```python
from build123d import *

# Parameters (mm, degrees)
SKETCH1_W              = 44
SKETCH1_H              = 8
BOSS_EXTRUDE1_DEPTH    = 5
SKETCH2_W              = 3.945665761
SKETCH2_H              = 8
BOSS_EXTRUDE2_DEPTH    = 17
SKETCH3_W              = 8
SKETCH3_H              = 3
BOSS_EXTRUDE3_DEPTH    = 15
SKETCH4_W              = 5.850643969
SKETCH4_H              = 8
BOSS_EXTRUDE4_DEPTH    = 12
SKETCH5_W              = 4
SKETCH5_H              = 8
BOSS_EXTRUDE5_DEPTH    = 8
FILLET2_R              = 4
LPATTERN1_COUNT        = 5
LPATTERN1_PITCH        = 10
FILLET2_OF_LPATTERN1_R = 4
SKETCH6_R              = 1.941337646
CUT_EXTRUDE1_DEPTH     = 67.452838302
SKETCH7_W              = 44
SKETCH7_H              = 5
BOSS_EXTRUDE6_DEPTH    = 4.5
SKETCH8_W              = 12.5
SKETCH8_H              = 5
BOSS_EXTRUDE7_DEPTH    = 4.5
SKETCH9_W              = 48.5
SKETCH9_H              = 5
BOSS_EXTRUDE8_DEPTH    = 4.5
SKETCH10_W             = 17
SKETCH10_H             = 5
BOSS_EXTRUDE9_DEPTH    = 4.5
FILLET4_R              = 3


with BuildPart() as part:
    # Sketch1 → Boss-Extrude1 (new body)
    with BuildSketch(Plane(origin=(0, 0, 0), x_dir=(1, 0, 0), z_dir=(0, 1, 0))):
        Rectangle(SKETCH1_W, SKETCH1_H)
    extrude(amount=BOSS_EXTRUDE1_DEPTH)

    # Sketch2 → Boss-Extrude2 (add)
    with BuildSketch(Plane(origin=(0, 5, 0), x_dir=(1, 0, 0), z_dir=(0, 1, 0))):
        with Locations((20.027167119, 0)):
            Rectangle(SKETCH2_W, SKETCH2_H)
    boss_extrude2 = extrude(amount=BOSS_EXTRUDE2_DEPTH)

    # Sketch3 → Boss-Extrude3 (add)
    with BuildSketch(Plane.ZY.offset(-18.054334239)):
        with Locations((0, 23.5)):
            Rectangle(SKETCH3_W, SKETCH3_H)
    boss_extrude3 = extrude(amount=-BOSS_EXTRUDE3_DEPTH)

    # Sketch4 → Boss-Extrude4 (add)
    with BuildSketch(Plane(origin=(0, 25, 0), x_dir=(1, 0, 0), z_dir=(0, 1, 0))):
        with Locations((30.129012255, 0)):
            Rectangle(SKETCH4_W, SKETCH4_H)
    boss_extrude4 = extrude(amount=BOSS_EXTRUDE4_DEPTH)

    # Mirror1: Boss-Extrude2, Boss-Extrude3, Boss-Extrude4 across plane
    add(boss_extrude2.mirror(Plane(origin=(0, 0, 0), x_dir=(0, 0, 1), z_dir=(1, 0, 0))))
    add(boss_extrude3.mirror(Plane(origin=(0, 0, 0), x_dir=(0, 0, 1), z_dir=(1, 0, 0))))
    add(boss_extrude4.mirror(Plane(origin=(0, 0, 0), x_dir=(0, 0, 1), z_dir=(1, 0, 0))))

    # Sketch5 → Boss-Extrude5 (add)
    with BuildSketch(Plane.XZ):
        with Locations((20, 0)):
            Rectangle(SKETCH5_W, SKETCH5_H)
    boss_extrude5 = extrude(amount=BOSS_EXTRUDE5_DEPTH)

    # Fillet2
    fillet2_edges = [part.edges().sort_by_distance(p)[0] for p in [
        (20, -8, -4),
        (20, -8, 4),
    ]]
    fillet(fillet2_edges, radius=FILLET2_R - 0.0001)  # a hair under: the kernel refuses the full size

    # LPattern1: Boss-Extrude5 ×5
    with Locations(*[(-i * LPATTERN1_PITCH, 0, 0) for i in range(1, LPATTERN1_COUNT)]):
        add(boss_extrude5)

    # Fillet2 of LPattern1
    fillet2_of_lpattern1_edges = [part.edges().sort_by_distance(p)[0] for p in [
        (10, -8, -4),
        (10, -8, 4),
        (0, -8, -4),
        (0, -8, 4),
        (-10, -8, -4),
        (-10, -8, 4),
        (-20, -8, -4),
        (-20, -8, 4),
    ]]
    fillet(fillet2_of_lpattern1_edges, radius=FILLET2_OF_LPATTERN1_R - 0.0001)  # a hair under: the kernel refuses the full size

    # Sketch6 → Cut-Extrude1 (cut, through all)
    with BuildSketch(Plane(origin=(22, 0, 0), x_dir=(0, 0, -1), z_dir=(1, 0, 0))):
        with Locations((0, -4)):
            Circle(SKETCH6_R)
    extrude(amount=-CUT_EXTRUDE1_DEPTH, mode=Mode.SUBTRACT)

    # Sketch7 → Boss-Extrude6 (add)
    with BuildSketch(Plane.XY.offset(4)):
        with Locations((0, 2.5)):
            Rectangle(SKETCH7_W, SKETCH7_H)
    extrude(amount=BOSS_EXTRUDE6_DEPTH)

    # Sketch8 → Boss-Extrude7 (add)
    with BuildSketch(Plane.ZY.offset(22)):
        with Locations((2.25, 2.5)):
            Rectangle(SKETCH8_W, SKETCH8_H)
    extrude(amount=BOSS_EXTRUDE7_DEPTH)

    # Sketch9 → Boss-Extrude8 (add)
    with BuildSketch(Plane(origin=(0, 0, -4), x_dir=(-1, 0, 0), z_dir=(0, 0, -1))):
        with Locations((2.25, 2.5)):
            Rectangle(SKETCH9_W, SKETCH9_H)
    extrude(amount=BOSS_EXTRUDE8_DEPTH)

    # Sketch10 → Boss-Extrude9 (add)
    with BuildSketch(Plane(origin=(22, 0, 0), x_dir=(0, 0, -1), z_dir=(1, 0, 0))):
        with Locations((0, 2.5)):
            Rectangle(SKETCH10_W, SKETCH10_H)
    extrude(amount=BOSS_EXTRUDE9_DEPTH)

    # Fillet4
    fillet4_edges = [part.edges().sort_by_distance(p)[0] for p in [
        (33.054334239, 22, 0),
        (18.054334239, 25, 0),
        (27.20369027, 25, 0),
        (-18.054334239, 25, 0),
        (-33.054334239, 22, 0),
        (-27.20369027, 25, 0),
    ]]
    fillet(fillet4_edges, radius=FILLET4_R)


solid = part.part
```
Source: CAD feature listing. Evaluate the final solid. Frame: model axes, mm. A direction names the side the tool comes from. Give positions to 0.01 mm unless a question says otherwise; leave off trailing zeros. Write each loop counter-clockwise with the first axis right and the second up, starting at its lowest first coordinate (ties: lowest second). Pieces come first, ordered by that corner, then holes.
1. Material intervals for line 1 along Y through (x, z) = (-10.3, 0); line 2 along X through (y, z) = (13, 2); line 3 along X through (y, z) = (2, -1.5), sorted ascending.
2. Section query A-A (y = 10). Return the cut outline in (x, z).
3. Pull-direction query (X, two-part tool) for faces 1 (the face through (-27.204, 32, 0)), 2 (the face through (-33.054, 31, 0)), 3 (the face through (0.028, -2.075, 0.253)); classes: +X half, -X half, draft (parallel to the pull), parting line (faces both ways), or undercut.
4. First-contact query: pin 1 (4 mm diameter, centred on y = 17, z = -2, fed in from -X); pin 2 (4 mm diameter, centred on x = -24.5, z = 1, fed in from -Y); pin 3 (2.5 mm diameter, centred on y = -3, z = 0.5, fed in from +X). Flat tips, straight axial feed; report the tip coordinate or a pass-through.
5. Access query for faces 4 (the face through (-10, -2, -4)), 5 (the face through (-26.5, 2, 0)), 6 (the face through (-2, -2, 1)), 7 (the face through (10, -2, 4)). Directions: +Z, -Z, +X, -X, +Y, -Y. A direction counts if a zero-diameter tool reaches every point of the face in a straight line with its end or side. Return the directions, or none.
6. Section query C-C (z = 5.75). Return the cut outline in (x, y).
Output values:
1. line 1: y = -8 to -5.94, -2.06 to 5
1. line 2: x = -22 to -18.05, 18.05 to 22
1. line 3: x = -26.5 to 26.5
2. outline: (-22, -4) - (-18.05, -4) - (-18.05, 4) - (-22, 4) - close; (18.05, -4) - (22, -4) - (22, 4) - (18.05, 4) - close
3. face 1: undercut
3. face 2: -X half
3. face 3: draft
4. pin 1: stops at x = -22
4. pin 2: stops at y = 0
4. pin 3: stops at x = 22
5. face 4: -Z, +X, -X, -Y
5. face 5: +Z, -Z, -X, -Y
5. face 6: +Z, -Z, -Y
5. face 7: +Z, +X, -X, -Y
6. outline: (-26.5, 0) - (26.5, 0) - (26.5, 5) - (-26.5, 5) - close
